```python
from build123d import *

# Parameters (mm, degrees)
SKETCH1_R               = 38.1
BOSS_EXTRUDE1_DEPTH     = 2.54
SKETCH2_R               = 38.1
SKETCH2_R_2             = 35.56
BOSS_EXTRUDE2_DEPTH     = 16.51
CUT_EXTRUDE1_REACH      = 89.298
CUT_EXTRUDE1_END_RADIUS = 35.56
SKETCH3_R               = 3.175


with BuildPart() as part:
    # Sketch1 → Boss-Extrude1 (new body)
    with BuildSketch(Plane(origin=(0, 0, 0), x_dir=(1, 0, 0), z_dir=(0, 1, 0))):
        with Locations(Location((0, 0, 0), (0, 0, 270))):
            Circle(SKETCH1_R)
    extrude(amount=BOSS_EXTRUDE1_DEPTH)

    # Sketch2 → Boss-Extrude2 (add)
    with BuildSketch(Plane(origin=(0, 2.54, 0), x_dir=(1, 0, 0), z_dir=(0, 1, 0))):
        with Locations(Location((0, 0, 0), (0, 0, 270))):
            Circle(SKETCH2_R)
        with Locations(Location((0, 0, 0), (0, 0, 270))):
            Circle(SKETCH2_R_2, mode=Mode.SUBTRACT)
    extrude(amount=BOSS_EXTRUDE2_DEPTH)

    # Cut-Extrude1: up to this cylinder (the profile starts outside it)
    cut_extrude1_end = Plane(origin=(0, 9.525, 0), z_dir=(0, -1, 0)) * Cylinder(CUT_EXTRUDE1_END_RADIUS, 250.716, mode=Mode.PRIVATE)
    # Sketch3 → Cut-Extrude1 (cut, up to the surface)
    with BuildSketch(Plane.ZY.offset(38.1), mode=Mode.PRIVATE) as cut_extrude1_sk1:
        with Locations((0, 9.525)):
            Circle(SKETCH3_R)
    cut_extrude1_tool1 = extrude(cut_extrude1_sk1.sketch, amount=-CUT_EXTRUDE1_REACH, mode=Mode.PRIVATE) - cut_extrude1_end
    add(cut_extrude1_tool1.solids().sort_by_distance((-38.1, 9.525, 0))[0], mode=Mode.SUBTRACT)


solid = part.part
```
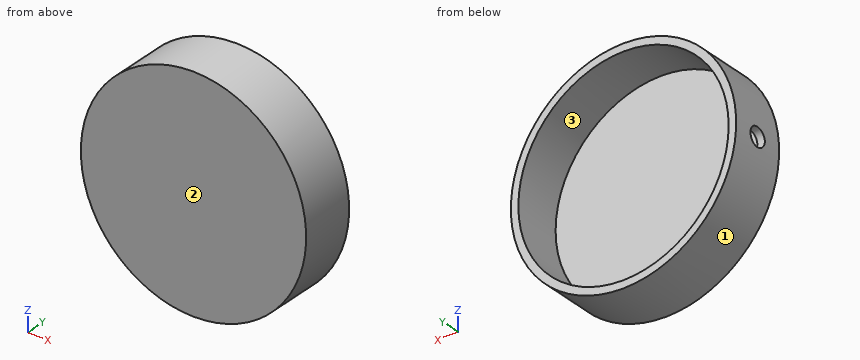
The listing builds one solid part. Answer for the finished solid, in the listing's coordinates (mm). Face numbers are marked on the shaded views. Coordinates: 2 decimals unless noted, no trailing zeros. Write each loop counter-clockwise with the first axis right and the second up, starting at its lowest first coordinate (ties: lowest second). Pieces come first, ordered by that corner, then holes. Notation, with made-up numbers: (-7.5, 24) - (2.5, 24) arc R6 ccw to (2.5, 35) - close; hole circle Ø3 at (28.25, -21.75). An arc over 180 degrees is marked (long way). Return JSON: item names as keys, results as strings. Group by question number.
Q1. For a pull along Z with two mould halves and no side action, classify the marked faces 1, 2 and 3 as +Z half, -Z half, draft (parallel to the pull), parting line (faces both ways), or undercut.
Q2. The part is cut by section A-A on z = 0. Write down the section's boundary in (x, y), and give its area (3 significant figures).
Q3. Flat-ended cylindrical pins translate along their axes: pin 1 Ø10 at (x, y) = (-6, 7.5) entering from +Z; pin 2 Ø5.5 at (y, z) = (9.525, 0) entering from +X; pin 3 Ø3 at (x, y) = (-24.5, 3) entering from +Z; pin 4 Ø1.5 at (x, z) = (-19.5, 29.5) entering from -Y. Find the tip coordinate at first contact, or state that the pin passes through.
Q4. The part is cut by section B-B on x = 0. Write down the section's boundary in (y, z), and give its area (3 significant figures).
Q5. Find the intervals of material crossed by line 1 along Y through (x, z) = (-36, 0); line 2 along X through (y, z) = (14.5, 0); line 3 along Y through (x, z) = (3, 4), in increasing order. Write a range as [from, to].
Q6. The part is cut by section D-D on x = -12.5. Write down the section's boundary in (y, z).
Q7. The part is cut by section C-C on y = 15.25. Write down the section's boundary in (x, z), and give its area (3 significant figures).
Evaluation:
{
 "1": {"face 1": "parting line", "face 2": "draft", "face 3": "undercut"},
 "2": {"outline": "(-38.1, 0) - (38.1, 0) - (38.1, 19.05) - (35.56, 19.05) - (35.56, 2.54) - (-35.56, 2.54) - (-35.56, 6.35) - (-38.1, 6.35) - close; (-38.1, 12.7) - (-35.56, 12.7) - (-35.56, 19.05) - (-38.1, 19.05) - close", "area": "261 mm2"},
 "3": {"pin 1": "stops at z = 38.09", "pin 2": "stops at x = 38.1", "pin 3": "stops at z = 30.37", "pin 4": "stops at y = 0"},
 "4": {"outline": "(0, -38.1) - (19.05, -38.1) - (19.05, -35.56) - (2.54, -35.56) - (2.54, 35.56) - (19.05, 35.56) - (19.05, 38.1) - (0, 38.1) - close", "area": "277 mm2"},
 "5": {"line 1": "y = [0, 6.35], [12.7, 19.05]", "line 2": "x = [-38.1, -35.56], [35.56, 38.1]", "line 3": "y = [0, 2.54]"},
 "6": {"outline": "(0, -35.99) - (19.05, -35.99) - (19.05, -33.29) - (2.54, -33.29) - (2.54, 33.29) - (19.05, 33.29) - (19.05, 35.99) - (0, 35.99) - close"},
 "7": {"outline": "circle Ø76.2 at (0, 0); hole circle Ø71.12 at (0, 0)", "area": "588 mm2"}
}
